Check sheet for the modelled part. Datum: model origin and axes. Units: mm. Face numbers are marked on the shaded views. A direction names the side the tool comes from. Coordinates: 2 decimals unless noted, no trailing zeros. Loops run counter-clockwise (first coordinate to the right, second up) from the corner with the lowest first, then second, coordinate; pieces in that order, holes last. Notation, with made-up numbers: (0.5, 82) - (13.5, 82) arc R28 cw to (13.5, 120) - close; hole circle Ø4 at (45, 82). An arc over 180 degrees is marked (long way). Use a Markdown table: item, result. Add a question column.
1) Sectioned sample at D-D, the plane y = 2. Enter the section's corners in (x, z).
2) Thickness scan on line 1 (X direction, y = 14.5, z = 2.25); line 2 (X direction, y = -10.5, z = -0.75); line 3 (Y direction, x = -1, z = -0.75). Record the ranges inside material, lowest first.
3) Tool access check on the marked faces 1, 2, 3, 4 and 5. Record the directions out of +Z, -Z, +X, -X, +Y, -Y that give a thin tool (end or side, any length) a straight path to the whole face; none if there is none.
4) Sectioned sample at A-A, the plane x = 5.5. Enter the section's corners in (y, z).
5) Draft check along X on the marked faces 6, 7, 8 and 9. Enter one of: pulls with the +X half, pulls with the -X half, needs draft (parallel to the pull), parting line crosses it, or undercut.
6) Sectioned sample at C-C, the plane y = -3.5. Enter the section's corners in (x, z).
7) Sectioned sample at B-B, the plane z = 3. Enter the section's corners in (x, y).
8) Go/stop test with flat-tipped pins: P1, Ø2.5, axis at x = 39, z = 3, coming from the +Y side; P2, Ø1.5, axis at x = -30, z = 4, coming from the +Y side; P3, Ø1.5, axis at y = -3.5, z = -4.5, coming from the -X side. Record where each tip stops, or that it passes through.
from build123d import *

# Parameters (mm, degrees)
F1_DEPTH = 6.35
F3_DEPTH = 12.701
F7_R     = 2.032


# Not quite as in the source:
# - a feature of the source that left no trace in its solid (it failed there, or was rolled back) is left out


with BuildPart() as f1:
    # F0 (on Top) → F1 (new body, symmetric)
    with BuildSketch(Plane.XY):
        with BuildLine():
            Line((16.3520683207, 8.89), (-16.3520683207, 8.89))
            ThreePointArc((-16.3520683207, 8.89), (-49.53, 0), (-16.3520683207, -8.89))
            Line((-16.3520683207, -8.89), (16.3520683207, -8.89))
            ThreePointArc((16.3520683207, -8.89), (49.53, 0), (16.3520683207, 8.89))
        make_face()
    extrude(amount=F1_DEPTH, both=True)

    # F4: F3 across plane


with BuildPart() as f3:
    # F2 (on face) → F3 (new body, through all)
    with BuildSketch(Plane.XY.offset(6.35)):
        Polygon((-35.5073561069, -8.89), (-30.3747122138, 0), (-35.5073561069, 8.89), (-45.7726438931, 8.89), (-49.53, 8.89), (-49.53, 0), (-49.53, -8.89), (-45.7726438931, -8.89), align=None)
    extrude(amount=-F3_DEPTH)


with BuildPart() as f1_1:
    add(f1.part)
    add(f3.part.mirror(Plane.YZ), mode=Mode.SUBTRACT)

    # F5: cut F3
    add(f3.part, mode=Mode.SUBTRACT)

    # F7
    f7_edges = [f1_1.edges().sort_by_distance(p)[0] for p in [
        (0, -8.89, 6.35),
        (-31.75, -17.78, 6.35),
        (-31.75, 17.78, 6.35),
        (0, 8.89, 6.35),
        (31.75, 17.78, 6.35),
        (31.75, -17.78, 6.35),
        (-31.75, -17.78, -6.35),
        (0, -8.89, -6.35),
        (31.75, -17.78, -6.35),
        (31.75, 17.78, -6.35),
        (0, 8.89, -6.35),
        (-31.75, 17.78, -6.35),
        (-16.352068, -8.89, 0),
        (16.352068, -8.89, 0),
        (-16.352068, 8.89, 0),
        (16.352068, 8.89, 0),
        (-47.147932, 8.89, 0),
        (47.147932, 8.89, 0),
        (47.147932, -8.89, 0),
        (-47.147932, -8.89, 0),
    ]]
    fillet(f7_edges, radius=F7_R)


solid = f1_1.part
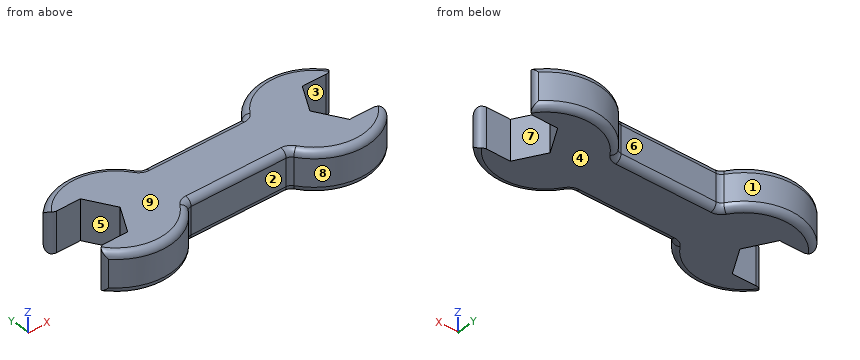
Solved:
| question | item | result |
|---|---|---|
| 1 | outline | (-31.53, -6.35) - (31.53, -6.35) - (31.53, 6.35) - (-31.53, 6.35) - close |
| 2 | line 1 | x = -42.04 to -21.46, 21.46 to 42.04 |
| 2 | line 2 | x = -45.08 to -17.4, 17.4 to 45.08 |
| 2 | line 3 | y = -8.89 to 8.89 |
| 3 | face 1 | +Z, -Z, +Y |
| 3 | face 2 | +Z, -Z, -Y |
| 3 | face 3 | +Z, -Z, +X |
| 3 | face 4 | -Z, +X, -X, +Y, -Y |
| 3 | face 5 | +Z, -Z, -X |
| 4 | outline | (-8.89, -4.32) arc R2.03 ccw to (-6.86, -6.35) - (6.86, -6.35) arc R2.03 ccw to (8.89, -4.32) - (8.89, 4.32) arc R2.03 ccw to (6.86, 6.35) - (-6.86, 6.35) arc R2.03 ccw to (-8.89, 4.32) - close |
| 5 | face 6 | undercut |
| 5 | face 7 | pulls with the +X half |
| 5 | face 8 | undercut |
| 5 | face 9 | needs draft |
| 6 | outline | (-32.4, -6.35) - (32.4, -6.35) - (32.4, 6.35) - (-32.4, 6.35) - close |
| 7 | outline | (-44.56, -12.33) arc R17.78 ccw to (-16.92, -9.8) arc R2.03 cw to (-15.22, -8.89) - (15.22, -8.89) arc R2.03 cw to (16.92, -9.8) arc R17.78 ccw to (44.56, -12.33) arc R2.03 ccw to (43.1, -8.89) - (35.51, -8.89) - (30.37, 0) - (35.51, 8.89) - (43.1, 8.89) arc R2.03 ccw to (44.56, 12.33) arc R17.78 ccw to (16.92, 9.8) arc R2.03 cw to (15.22, 8.89) - (-15.22, 8.89) arc R2.03 cw to (-16.92, 9.8) arc R17.78 ccw to (-44.56, 12.33) arc R2.03 ccw to (-43.1, 8.89) - (-35.51, 8.89) - (-30.37, 0) - (-35.51, -8.89) - (-43.1, -8.89) arc R2.03 ccw to start |
| 8 | P1 | stops at y = 16.74 |
| 8 | P2 | stops at y = 17.75 |
| 8 | P3 | stops at x = -32.83 |
